The listing builds one solid part. Answer for the finished solid, in the listing's coordinates (mm). Coordinates: 2 decimals unless noted, no trailing zeros. Order: outer loops, then holes, each group sorted by start corner. A loop starts at its lowest first (then second) coordinate and runs counter-clockwise, first axis right, second up.
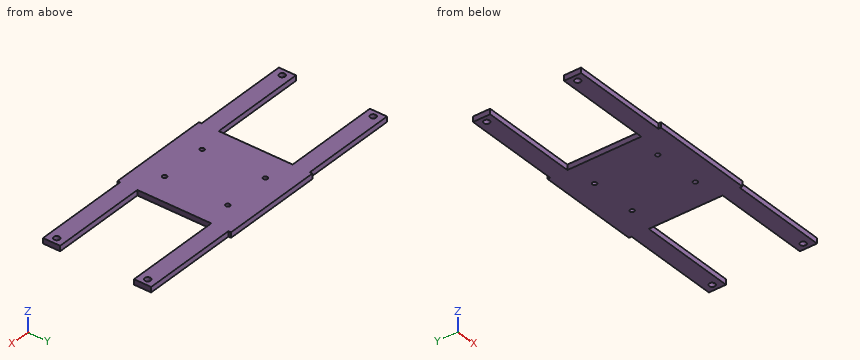
```python
from build123d import *

# Parameters (mm, degrees)
SENSOR_BRIDGE_DEPTH      = 4
DECK_COLUMNS_M4_START    = -1
SKETCH_DECK_COLUMNS_M4_R = 2.25
DECK_COLUMNS_M4_DEPTH    = 6
MID360_MOUNT_START       = -1
SKETCH_MID360_MOUNT_R    = 1.65
MID360_MOUNT_DEPTH       = 6


with BuildPart() as part:
    # Sketch_Sensor_bridge → Sensor_bridge (new body)
    with BuildSketch(Plane.XY):
        Polygon((113, -28), (113, -41), (39, -41), (39, -43), (-39, -43), (-39, -41), (-113, -41), (-113, -28), (-39, -28), (-39, 28), (-113, 28), (-113, 41), (-39, 41), (-39, 43), (39, 43), (39, 41), (113, 41), (113, 28), (39, 28), (39, -28), align=None)
    extrude(amount=SENSOR_BRIDGE_DEPTH)

    # Sketch_Deck_columns_M4 → Deck_columns_M4 (cut)
    with BuildSketch(Plane.XY.offset(DECK_COLUMNS_M4_START)):
        with Locations(Location((-108, -34.5, 0), (0, 0, 180))):
            Circle(SKETCH_DECK_COLUMNS_M4_R)
        with Locations(Location((-108, 34.5, 0), (0, 0, 180))):
            Circle(SKETCH_DECK_COLUMNS_M4_R)
        with Locations(Location((108, -34.5, 0), (0, 0, 180))):
            Circle(SKETCH_DECK_COLUMNS_M4_R)
        with Locations(Location((108, 34.5, 0), (0, 0, 180))):
            Circle(SKETCH_DECK_COLUMNS_M4_R)
    extrude(amount=DECK_COLUMNS_M4_DEPTH, mode=Mode.SUBTRACT)

    # Sketch_MID360_mount → MID360_mount (cut)
    with BuildSketch(Plane.XY.offset(MID360_MOUNT_START)):
        with Locations(Location((-18, -24, 0), (0, 0, 180))):
            Circle(SKETCH_MID360_MOUNT_R)
        with Locations(Location((-18, 24, 0), (0, 0, 180))):
            Circle(SKETCH_MID360_MOUNT_R)
        with Locations(Location((18, -24, 0), (0, 0, 180))):
            Circle(SKETCH_MID360_MOUNT_R)
        with Locations(Location((18, 24, 0), (0, 0, 180))):
            Circle(SKETCH_MID360_MOUNT_R)
    extrude(amount=MID360_MOUNT_DEPTH, mode=Mode.SUBTRACT)


solid = part.part
```
(1) Each of these flat-tipped pins is pushed along its axis until it touches: pin 1 Ø2 at (x, z) = (-77, 1.5) entering from +Y; pin 2 Ø2 at (y, z) = (-42.5, 2.5) entering from -X; pin 3 Ø1.2 at (x, z) = (-66.5, 1) entering from -Y. Where does it stop, or does it pass through?
(2) Find section C-C (y = -8). Write down the section's boundary in (x, z).
(3) Find section B-B (z = 3.2). Give the number of separate pieces and of enclosed holes in the cut face, and give its area (3 significant figures).
(4) Find section A-A (x = -108). Write down the section's boundary in (y, z).
(5) Consider line 1 (Y direction, x = 72, z = 0.55); line 2 (Y direction, x = -18, z = 1.35); line 3 (X direction, y = 34, z = 2.7). Determine where each line is inside the solid, lowest interval first.
Findings below:
1. pin 1: stops at y = 41
1. pin 2: stops at x = -39
1. pin 3: stops at y = -41
2. outline: (-39, 0) - (39, 0) - (39, 4) - (-39, 4) - close
3. separate pieces: 1
3. enclosed holes: 8
3. area: 10,500 mm2
4. outline: (-41, 0) - (-36.75, 0) - (-36.75, 4) - (-41, 4) - close; (-32.25, 0) - (-28, 0) - (-28, 4) - (-32.25, 4) - close; (28, 0) - (32.25, 0) - (32.25, 4) - (28, 4) - close; (36.75, 0) - (41, 0) - (41, 4) - (36.75, 4) - close
5. line 1: y = -41 to -28, 28 to 41
5. line 2: y = -43 to -25.65, -22.35 to 22.35, 25.65 to 43
5. line 3: x = -113 to -110.19, -105.81 to 105.81, 110.19 to 113
